CAD build for the part. Positions are in the model's coordinates, mm. Face numbers are marked on the shaded views. Round coordinates to 2 decimals unless told otherwise and drop trailing zeros. Loops run counter-clockwise (first coordinate to the right, second up) from the corner with the lowest first, then second, coordinate; pieces in that order, holes last.
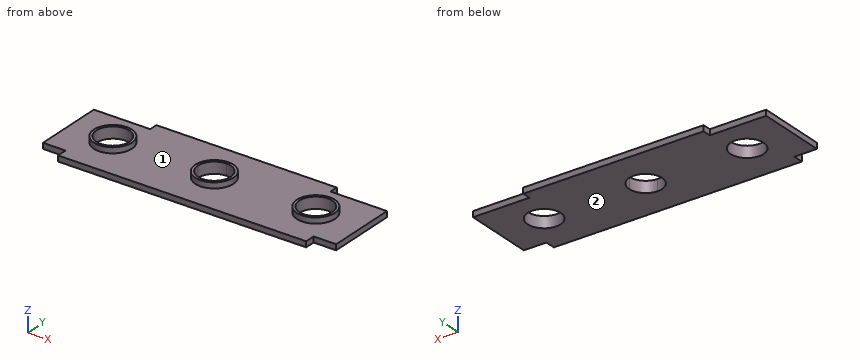
from build123d import *

# Parameters (mm, degrees)
F0_R     = 85.725
F1_DEPTH = 25.4
F0_R_2   = 74.1873427713
F2_DEPTH = 50.8
F3_DEPTH = 50.8
F4_DEPTH = 50.8


with BuildPart() as f1:
    # F0 (on Top) → F1 (new body)
    with BuildSketch(Plane.XY):
        with BuildLine():
            Line((193.6448768675, 306.0437094688), (-60.3551231325, 306.0437094688))
            Line((-60.3551231325, 306.0437094688), (-60.3551231325, -8.2812905312))
            Line((-60.3551231325, -8.2812905312), (41.2448768675, -8.2812905312))
            Line((41.2448768675, -8.2812905312), (41.2448768675, -54.3187905312))
            Line((41.2448768675, -54.3187905312), (600.0448768675, -54.3187905312))
            Line((600.0448768675, -54.3187905312), (600.0448768675, 59.1874594688))
            ThreePointArc((600.0448768675, 59.1874594688), (539.4281480503, 84.2957306516), (514.3198768675, 144.9124594688))
            ThreePointArc((514.3198768675, 144.9124594688), (539.4281480503, 205.5291882861), (600.0448768675, 230.6374594688))
            Line((600.0448768675, 230.6374594688), (600.0448768675, 344.1437094688))
            Line((600.0448768675, 344.1437094688), (193.6448768675, 344.1437094688))
            Line((193.6448768675, 344.1437094688), (193.6448768675, 306.0437094688))
        make_face()
        with Locations((142.8448768675, 144.9124594688)):
            Circle(F0_R, mode=Mode.SUBTRACT)
        with BuildLine():
            Line((1006.4448768675, 344.1437094688), (600.0448768675, 344.1437094688))
            Line((600.0448768675, 344.1437094688), (600.0448768675, 230.6374594688))
            ThreePointArc((600.0448768675, 230.6374594688), (660.6616056848, 205.5291882861), (685.7698768675, 144.9124594688))
            ThreePointArc((685.7698768675, 144.9124594688), (660.6616056848, 84.2957306516), (600.0448768675, 59.1874594688))
            Line((600.0448768675, 59.1874594688), (600.0448768675, -54.3187905312))
            Line((600.0448768675, -54.3187905312), (1158.8448768675, -54.3187905312))
            Line((1158.8448768675, -54.3187905312), (1158.8448768675, -8.2812905312))
            Line((1158.8448768675, -8.2812905312), (1260.4448768675, -8.2812905312))
            Line((1260.4448768675, -8.2812905312), (1260.4448768675, 306.0437094688))
            Line((1260.4448768675, 306.0437094688), (1006.4448768675, 306.0437094688))
            Line((1006.4448768675, 306.0437094688), (1006.4448768675, 344.1437094688))
        make_face()
        with BuildLine():
            ThreePointArc((1142.9698768675, 144.9124594688), (1057.2448768675, 59.1874594688), (971.5198768675, 144.9124594688))
            ThreePointArc((971.5198768675, 144.9124594688), (1057.2448768675, 230.6374594688), (1142.9698768675, 144.9124594688))
        make_face(mode=Mode.SUBTRACT)
    extrude(amount=F1_DEPTH)

    # F0 (on Top) → F2 (join)
    with BuildSketch(Plane.XY):
        with Locations((142.8448768675, 144.9124594688)):
            Circle(F0_R)
        with Locations((142.8448768675, 144.9124594688)):
            Circle(F0_R_2, mode=Mode.SUBTRACT)
    extrude(amount=F2_DEPTH)

    # F0 (on Top) → F3 (join)
    with BuildSketch(Plane.XY):
        with BuildLine():
            Line((600.0448768675, 71.2306225134), (600.0448768675, 59.1874594688))
            ThreePointArc((600.0448768675, 59.1874594688), (660.6616056848, 84.2957306516), (685.7698768675, 144.9124594688))
            Line((685.7698768675, 144.9124594688), (673.726713823, 144.9124594688))
            ThreePointArc((673.726713823, 144.9124594688), (652.145803429, 92.8115329074), (600.0448768675, 71.2306225134))
        make_face()
        with BuildLine():
            ThreePointArc((685.7698768675, 144.9124594688), (660.6616056848, 205.5291882861), (600.0448768675, 230.6374594688))
            Line((600.0448768675, 230.6374594688), (600.0448768675, 218.5942964243))
            ThreePointArc((600.0448768675, 218.5942964243), (652.145803429, 197.0133860303), (673.726713823, 144.9124594688))
            Line((673.726713823, 144.9124594688), (685.7698768675, 144.9124594688))
        make_face()
        with BuildLine():
            Line((600.0448768675, 218.5942964243), (600.0448768675, 230.6374594688))
            ThreePointArc((600.0448768675, 230.6374594688), (539.4281480503, 205.5291882861), (514.3198768675, 144.9124594688))
            Line((514.3198768675, 144.9124594688), (526.3630399121, 144.9124594688))
            ThreePointArc((526.3630399121, 144.9124594688), (547.9439503061, 197.0133860303), (600.0448768675, 218.5942964243))
        make_face()
        with BuildLine():
            ThreePointArc((514.3198768675, 144.9124594688), (539.4281480503, 84.2957306516), (600.0448768675, 59.1874594688))
            Line((600.0448768675, 59.1874594688), (600.0448768675, 71.2306225134))
            ThreePointArc((600.0448768675, 71.2306225134), (547.9439503061, 92.8115329074), (526.3630399121, 144.9124594688))
            Line((526.3630399121, 144.9124594688), (514.3198768675, 144.9124594688))
        make_face()
    extrude(amount=F3_DEPTH)

    # F0 (on Top) → F4 (join)
    with BuildSketch(Plane.XY):
        with BuildLine():
            ThreePointArc((1142.9698768675, 144.9124594688), (1057.2448768675, 230.6374594688), (971.5198768675, 144.9124594688))
            ThreePointArc((971.5198768675, 144.9124594688), (1057.2448768675, 59.1874594688), (1142.9698768675, 144.9124594688))
        make_face()
        with BuildLine():
            ThreePointArc((1131.6165984788, 144.9124594688), (1057.2448768675, 70.5407378575), (982.8731552562, 144.9124594688))
            ThreePointArc((982.8731552562, 144.9124594688), (1057.2448768675, 219.2841810801), (1131.6165984788, 144.9124594688))
        make_face(mode=Mode.SUBTRACT)
    extrude(amount=F4_DEPTH)


solid = f1.part
Item 1: Cut at B-B (y = 162.5). List the corners of the cut face in (x, z).
Verdict:
outline: (-60.36, 0) - (70.77, 0) - (70.77, 50.8) - (58.94, 50.8) - (58.94, 25.4) - (-60.36, 25.4) - close; (214.92, 0) - (528.49, 0) - (528.49, 50.8) - (516.14, 50.8) - (516.14, 25.4) - (226.75, 25.4) - (226.75, 50.8) - (214.92, 50.8) - close; (671.6, 0) - (984.98, 0) - (984.98, 50.8) - (973.34, 50.8) - (973.34, 25.4) - (683.95, 25.4) - (683.95, 50.8) - (671.6, 50.8) - close; (1129.51, 0) - (1260.44, 0) - (1260.44, 25.4) - (1141.15, 25.4) - (1141.15, 50.8) - (1129.51, 50.8) - close
Item 2: Wall check: L1, parallel to X at y = 160, z = 31; L2, parallel to X at y = 177.5, z = 23; L3, parallel to X at y = 94.5, z = 35. Give the ranges that are in metal, low to high.
Verdict:
L1: x = 58.46 to 70.21, 215.48 to 227.23, 515.66 to 527.92, 672.17 to 684.43, 972.86 to 984.42, 1130.07 to 1141.63
L2: x = -60.36 to 76.2, 209.49 to 533.96, 666.13 to 990.39, 1124.1 to 1260.44
L3: x = 73.51 to 88.42, 197.27 to 212.18, 530.71 to 546.31, 653.78 to 669.38, 987.91 to 1002.57, 1111.92 to 1126.58
Item 3: Cut at C-C (x = 656). List the corners of the cut face in (y, z).
Verdict:
outline: (-54.32, 0) - (96.97, 0) - (96.97, 50.8) - (79.97, 50.8) - (79.97, 25.4) - (-54.32, 25.4) - close; (192.85, 0) - (344.14, 0) - (344.14, 25.4) - (209.86, 25.4) - (209.86, 50.8) - (192.85, 50.8) - close
Item 4: Flat gauge pins, fed straight in: P1, Ø12, axis at x = 612, z = 40.5, coming from the +Y side; P2, Ø3, axis at y = 66, z = 43.5, coming from the -X side; P3, Ø20.5, axis at x = -32.5, z = 6.5, coming from the -Y side. Where does each tip first touch, or does it go through?
Verdict:
P1: stops at y = 230.43
P2: stops at x = 106.02
P3: stops at y = -8.28
Item 5: Mould opens along X. For the marked faces 1 and 2 say: released by +X, released by -X, zero draft, split by the parting line, or undercut.
Verdict:
face 1: undercut
face 2: zero draft
Item 6: Cut at A-A (z = 41). List the corners of the cut face in (x, y) (3 decimals), plus the area to 3 significant figures.
Verdict:
outline: circle Ø171.45 at (142.845, 144.912); circle Ø171.45 at (600.045, 144.912); circle Ø171.45 at (1057.245, 144.912); hole circle Ø148.375 at (142.845, 144.912); hole circle Ø147.364 at (600.045, 144.912); hole circle Ø148.743 at (1057.245, 144.912)
area: 17,500 mm2
Item 7: Cut at D-D (x = 1180). List the corners of the cut face in (y, z).
Verdict:
outline: (-8.28, 0) - (306.04, 0) - (306.04, 25.4) - (-8.28, 25.4) - close
